```python
from build123d import *

# Parameters (mm, degrees)
SKETCH_W        = 80
SKETCH_H        = 35
PAD_DEPTH       = 17
SKETCH001_W     = 52
SKETCH001_H     = 26
POCKET_DEPTH    = 13
SKETCH002_W     = 10
SKETCH002_H     = 5
POCKET001_DEPTH = 10
SKETCH005_R     = 5.25
POCKET004_DEPTH = 3
SKETCH007_W     = 20
SKETCH007_H     = 22
POCKET005_DEPTH = 12
SKETCH008_R     = 3.25
POCKET006_DEPTH = 6.5
CHAMFER_SIZE    = 1
CHAMFER001_SIZE = 1


with BuildPart() as part:
    # Sketch → Pad (new body)
    with BuildSketch(Plane.XY):
        with Locations((40, 17.5)):
            Rectangle(SKETCH_W, SKETCH_H)
    extrude(amount=PAD_DEPTH)

    # Sketch001 (on Face6 of Pad) → Pocket (cut)
    with BuildSketch(Plane.XY.offset(17)):
        with Locations((31, 17.5)):
            Rectangle(SKETCH001_W, SKETCH001_H)
    extrude(amount=-POCKET_DEPTH, mode=Mode.SUBTRACT)

    # Sketch002 (on Face2 of Pocket) → Pocket001 (cut)
    with BuildSketch(Plane(origin=(0, 0, 0), x_dir=(0, -1, 0), z_dir=(-1, 0, 0))):
        with Locations((-17.5, 9.5)):
            Rectangle(SKETCH002_W, SKETCH002_H)
    extrude(amount=-POCKET001_DEPTH, mode=Mode.SUBTRACT)

    # Sketch005 → Pocket004 (cut)
    with BuildSketch(Plane.XY.offset(4)):
        with Locations((15, 17.5)):
            Circle(SKETCH005_R)
        with Locations((45, 17.5)):
            Circle(SKETCH005_R)
    extrude(amount=-POCKET004_DEPTH, mode=Mode.SUBTRACT)

    # Sketch007 (on Face5 of Pocket004) → Pocket005 (cut)
    with BuildSketch(Plane.XY.offset(17)):
        with Locations((67, 17.5)):
            Rectangle(SKETCH007_W, SKETCH007_H)
    extrude(amount=-POCKET005_DEPTH, mode=Mode.SUBTRACT)

    # Sketch008 (on Face6 of Pocket005) → Pocket006 (cut)
    with BuildSketch(Plane(origin=(0, 35, 0), x_dir=(-1, 0, 0), z_dir=(0, 1, 0))):
        with Locations((-67, 10)):
            Circle(SKETCH008_R)
    extrude(amount=-POCKET006_DEPTH, mode=Mode.SUBTRACT)

    # Chamfer
    chamfer_edges = [part.edges().sort_by_distance(p)[0] for p in [
        (70.25, 28.5, 10),
    ]]
    chamfer(chamfer_edges, length=CHAMFER_SIZE)

    # Chamfer001
    chamfer001_edges = [part.edges().sort_by_distance(p)[0] for p in [
        (0, 22.5, 9.5),
        (0, 17.5, 7),
        (0, 17.5, 12),
        (0, 12.5, 9.5),
    ]]
    chamfer(chamfer001_edges, length=CHAMFER001_SIZE)


solid = part.part
```
For this review, take the finished solid that the model builds, in its own axes (mm). A direction names the side the tool comes from. Coordinates: 2 decimals unless noted, no trailing zeros. Write each loop counter-clockwise with the first axis right and the second up, starting at its lowest first coordinate (ties: lowest second). Pieces come first, ordered by that corner, then holes. Notation, with made-up numbers: (47.5, -36.75) -> (60.5, -36.75) arc R7 cw to (60.5, -27.75) -> close; hole circle Ø7 at (-36.5, 21.25). An arc over 180 degrees is marked (long way). Put each result on its own line as item: value.
Q1. Take a section at D-D, the plane x = 67. State the section outline as (y, z) points, then the cut area to 3 significant figures.
From the geometry:
outline: (0, 0) -> (35, 0) -> (35, 6.75) -> (29.5, 6.75) -> (28.5, 5.75) -> (28.5, 5) -> (6.5, 5) -> (6.5, 17) -> (0, 17) -> close; (28.5, 14.25) -> (29.5, 13.25) -> (35, 13.25) -> (35, 17) -> (28.5, 17) -> close
area: 288 mm2
Q2. Take a section at B-B, the plane z = 2.25. State the section outline as (x, y) points, then the cut area to 3 significant figures.
From the geometry:
outline: (0, 0) -> (80, 0) -> (80, 35) -> (0, 35) -> close; hole circle Ø10.5 at (15, 17.5); hole circle Ø10.5 at (45, 17.5)
area: 2,630 mm2
Q3. The part is to be moulded in two halves that separate along Y. For faces 1 (the flat face through (39, 35, 8)), 2 (the flat face through (39, 18, 0)), 3 (the flat face through (31, 30.5, 11)), 4 (the flat face through (39, 0, 8)), say which applies: +Y half, -Y half, draft (parallel to the pull), parting line (faces both ways), or undercut.
From the geometry:
face 1: +Y half
face 2: draft
face 3: undercut
face 4: -Y half
Q4. Tool access review of faces 5 (the cylindrical face through (40.83, 14.31, 2.52)), 6 (the flat face through (80, 17, 8)), 7 (the flat face through (3, 18, 7)): name each direction out of +Z, -Z, +X, -X, +Y, -Y from which nothing blocks a thin tool from reaching the whole face with its end or side.
From the geometry:
face 5: +Z
face 6: +Z, -Z, +X, +Y, -Y
face 7: -X
Q5. Take a section at A-A, the plane y = 19. State the section outline as (x, z) points.
From the geometry:
outline: (0, 0) -> (80, 0) -> (80, 17) -> (77, 17) -> (77, 5) -> (57, 5) -> (57, 4) -> (50.03, 4) -> (50.03, 1) -> (39.97, 1) -> (39.97, 4) -> (20.03, 4) -> (20.03, 1) -> (9.97, 1) -> (9.97, 4) -> (5, 4) -> (5, 7) -> (1, 7) -> (0, 6) -> close; (0, 13) -> (1, 12) -> (5, 12) -> (5, 17) -> (0, 17) -> close
Q6. Clearance check with flat-ended pins moving along their axes: pin 1 Ø3 at (x, y) = (16.5, 18) entering from +Z; pin 2 Ø4 at (x, y) = (49, 4) entering from -Z; pin 3 Ø13.5 at (x, y) = (45, 17.5) entering from +Z; pin 4 Ø6 at (x, z) = (67, 10) entering from +Y. State where each tip first meets the part, or that it passes through.
From the geometry:
pin 1: stops at z = 1
pin 2: stops at z = 0
pin 3: stops at z = 4
pin 4: stops at y = 6.5
Q7. Take a section at C-C, the plane x = 23. State the section outline as (y, z) points.
From the geometry:
outline: (0, 0) -> (35, 0) -> (35, 17) -> (30.5, 17) -> (30.5, 4) -> (4.5, 4) -> (4.5, 17) -> (0, 17) -> close
Q8. Wall thickness on L1, parallel to X at y = 12, z = 15; L2, parallel to Z at x = 67, y = 32.7; L3, parallel to Y at x = 15, z = 2.8: over which ranges is each line inside the solid? List them lowest first.
From the geometry:
L1: x = 0 to 5, 77 to 80
L2: z = 0 to 6.75, 13.25 to 17
L3: y = 0 to 12.25, 22.75 to 35
